Can you work these out from the model? Positions are in its coordinate system, mm. A direction names the side the tool comes from. Give positions to 0.01 mm unless a question says otherwise; leave off trailing zeros. Order: outer loops, then holes, each group sorted by start corner. A loop starts at its lowest first (then second) coordinate and runs counter-clockwise, first axis right, second up. Notation, with made-up numbers: M 24,69.25 L 43,69.25 A12 ccw 43,87.25 Z; hole C 60.25,59.25 d11. An arc over 180 degrees is marked long. Answer as a JSON object with one key per item and string values.
```python
from build123d import *

# Parameters (mm, degrees)
REVOLVE2_ANGLE      = 180
SKETCH4_W           = 20.32
SKETCH4_H           = 20.32
CUT_EXTRUDE2_DEPTH  = 32.004
BOSS_EXTRUDE2_DEPTH = 2.54
SKETCH5_W           = 2.54
SKETCH5_H           = 12.7
SKETCH5_W_2         = 12.7
SKETCH5_H_2         = 2.54
CUT_EXTRUDE3_DEPTH  = 2.54


with BuildPart() as part:
    # Sketch2 → Revolve2 (revolve)
    with BuildSketch(Plane.XY):
        Polygon((0, 0), (0, 40.64), (0, 45.63872), (25.4, 45.63872), (177.8, 52.292647699), (190.5, 52.292647699), (190.5, 47.293927699), (177.8, 47.293927699), (25.4, 40.64), (4.99872, 40.64), (4.99872, 0), align=None)
    revolve(axis=Axis((0, 0, 0), (1, 0, 0)), revolution_arc=REVOLVE2_ANGLE)

    # Sketch4 → Cut-Extrude2 (cut)
    with BuildSketch(Plane.ZY):
        with Locations((10.16, 10.16)):
            Rectangle(SKETCH4_W, SKETCH4_H)
        with Locations((10.16, -10.16)):
            Rectangle(SKETCH4_W, SKETCH4_H)
    extrude(amount=-CUT_EXTRUDE2_DEPTH, mode=Mode.SUBTRACT)

    # Sketch6 → Boss-Extrude2 (add)
    with BuildSketch(Plane(origin=(190.5, 0, 0), x_dir=(0, 0, -1), z_dir=(1, 0, 0))):
        with BuildLine():
            Line((-3.81, 50.911637334), (-3.81, 48.371637334))
            ThreePointArc((-3.81, 48.371637334), (-48.52145297, 0), (-3.81, -48.371637334))
            Line((-3.81, -48.371637334), (-3.81, -50.911637334))
            ThreePointArc((-3.81, -50.911637334), (-51.054, 0), (-3.81, 50.911637334))
        make_face()
    extrude(amount=BOSS_EXTRUDE2_DEPTH)

    # Sketch5 → Cut-Extrude3 (cut)
    with BuildSketch(Plane(origin=(0, 0, 0), x_dir=(-1, 0, 0), z_dir=(0, 0, -1))):
        with Locations((-2.49936, 34.29)):
            Rectangle(SKETCH5_W, SKETCH5_H)
        Polygon((-152.4, 49.954299749), (-152.4, 47.414299749), (-50.8, 42.97834795), (-50.8, 45.51834795), align=None)
        with Locations((-11.34872, 43.13936)):
            Rectangle(SKETCH5_W_2, SKETCH5_H_2)
        Polygon((-50.8, -42.97834795), (-50.8, -45.51834795), (-152.4, -49.954299749), (-152.4, -47.414299749), align=None)
        with Locations((-11.34872, -43.13936)):
            Rectangle(SKETCH5_W_2, SKETCH5_H_2)
        with Locations((-2.49936, -34.29)):
            Rectangle(SKETCH5_W, SKETCH5_H)
    extrude(amount=-CUT_EXTRUDE3_DEPTH, mode=Mode.SUBTRACT)


solid = part.part
```
1) I need wall thicknesses on L1, parallel to Y at x = 47.5, z = 10; L2, parallel to X at y = -31, z = 25.5; L3, parallel to Y at x = 145.5, z = 35. Which ranges of each line are inside material? Lowest first, please.
Results found:
{"L1": "y = -45.52 to -40.39, 40.39 to 45.52", "L2": "x = 0 to 5", "L3": "y = -36.93 to -29.67, 29.67 to 36.93"}
2) I want a section at D-D on x = 160. Write out the boundary of the cut face in (y, z).
Results found:
{"outline": "M -51.52,0 L -46.52,0 A46.52 cw 46.52,0 L 51.52,0 A51.52 ccw Z"}
3) I want a section at A-A on x = 131.5. Write out the boundary of the cut face in (y, z), and give its area (3 significant figures).
Results found:
{"outline": "M -50.27,0 L -49.04,0 L -49.04,2.54 L -46.5,2.54 L -46.5,0 L -45.27,0 A45.27 cw 45.27,0 L 46.5,0 L 46.5,2.54 L 49.04,2.54 L 49.04,0 L 50.27,0 A50.27 ccw Z", "area": "737 mm²"}
4) For faces 1 (the face through (102.311, -45.227, 1.252)), 2 (the face through (191.752, -1.069, 51.043)), 3 (the face through (191.75, 1.01, 48.51)), 4 (the face through (2, 20.32, 10)), which set-ups out of +Z, -Z, +X, -X, +Y, -Y let a thin tool reach every point of the face, with its end or its side?
Results found:
{"face 1": "-Z", "face 2": "+Z, +X", "face 3": "-Z, +X", "face 4": "-Z, +X, -X"}
5) I want a section at B-B on y = 0. Write out the boundary of the cut face in (x, z), and give its area (3 significant figures).
Results found:
{"outline": "M 0,20.32 L 5,20.32 L 5,40.64 L 25.4,40.64 L 177.8,47.29 L 190.5,47.29 L 190.5,48.52 L 193.04,48.52 L 193.04,51.05 L 190.5,51.05 L 190.5,52.29 L 177.8,52.29 L 25.4,45.64 L 0,45.64 Z", "area": "1,060 mm²"}
6) I want a section at C-C on x = 62.5. Write out the boundary of the cut face in (y, z), and give its area (3 significant figures).
Results found:
{"outline": "M -47.26,0 L -46.03,0 L -46.03,2.54 L -43.49,2.54 L -43.49,0 L -42.26,0 A42.26 cw 42.26,0 L 43.49,0 L 43.49,2.54 L 46.03,2.54 L 46.03,0 L 47.26,0 A47.26 ccw Z", "area": "690 mm²"}
7) I'm going to push flat-ended pins straight in: pin 1 Ø1 at (x, z) = (123.5, 42.5) entering from +Y; pin 2 Ø2 at (x, z) = (43.5, 33.5) entering from -Y; pin 3 Ø0.8 at (x, z) = (10, 1) entering from +Y; pin 4 Ø0.8 at (y, z) = (43, 1) entering from -X. Where does each tip first touch, or does it pass through?
Results found:
{"pin 1": "stops at y = 26.99", "pin 2": "stops at y = -33.16", "pin 3": "stops at y = 45.63", "pin 4": "stops at x = 0"}
8) Thinking about a two-plate mould opening in Y: for faces 5 (the face through (81.6, -43.3, 0)), 6 (the face through (15.06, 0.89, 40.63)), 7 (the face through (100.53, 0.97, 43.91)), 8 (the face through (12.878, 1.004, 45.628)), which applies, pulls with the +Y half, pulls with the -Y half, needs draft (parallel to the pull), parting line crosses it, or undercut?
Results found:
{"face 5": "needs draft", "face 6": "undercut", "face 7": "undercut", "face 8": "parting line crosses it"}
